Geometry: final body of the model. Coordinates: model frame, mm. A direction names the side the tool comes from. Round coordinates to 2 decimals unless told otherwise and drop trailing zeros. Write each loop counter-clockwise with the first axis right and the second up, starting at its lowest first coordinate (ties: lowest second). Pieces come first, ordered by that corner, then holes. Notation, with made-up numbers: M 75,37.5 L 128,37.5 A27 ccw 128,54.5 Z; hole C 47.25,42.25 d9. An arc over 180 degrees is marked long. Put each result on its own line as item: value. Start each with the question number.
```python
from build123d import *

# Parameters (mm, degrees)
SKETCH1_W            = 56
SKETCH1_H            = 199.6
EXTRUDE1_DEPTH       = 10
CHAMFER1_SIZE        = 1.5
HOLEWZD1_D           = 4
HOLEWZD1_DEPTH       = 5
HOLEWZD4_D           = 6.6
HOLEWZD4_DEPTH       = 10
HOLEWZD5_D           = 4
HOLEWZD5_DEPTH       = 10
HOLEWZD6_D           = 4
HOLEWZD6_DEPTH       = 5
HOLEWZD7_D           = 3.3
HOLEWZD9_D           = 4.5
HOLEWZD9_CBORE_D     = 8
HOLEWZD9_CBORE_DEPTH = 5


with BuildPart() as part:
    # Sketch1 → Extrude1 (new body)
    with BuildSketch(Plane.XY):
        with Locations((0, 78.3)):
            Rectangle(SKETCH1_W, SKETCH1_H)
    extrude(amount=EXTRUDE1_DEPTH)

    # Chamfer1
    chamfer1_edges = [part.edges().sort_by_distance(p)[0] for p in [
        (28, 78.3, 10),
        (0, 178.1, 10),
        (-28, 78.3, 10),
        (0, 178.1, 0),
        (28, 78.3, 0),
        (0, -21.5, 0),
        (-28, 78.3, 0),
        (0, -21.5, 10),
        (-28, 178.1, 5),
        (28, 178.1, 5),
        (28, -21.5, 5),
        (-28, -21.5, 5),
    ]]
    chamfer(chamfer1_edges, length=CHAMFER1_SIZE)

    # HoleWzd1
    with Locations(Plane(origin=(-28, 98.3, 0), x_dir=(-1, 0, 0), z_dir=(0, 0, -1))):
        with Locations((-40, -108.3), (-16, -108.3), (-40, 68.3), (-16, 68.3)):
            Hole(HOLEWZD1_D / 2, depth=HOLEWZD1_DEPTH)

    # HoleWzd4
    with Locations(Plane(origin=(0, 0, 0), x_dir=(-1, 0, 0), z_dir=(0, 0, -1))):
        with Locations((-12.5, 99.196924858), (12.5, 124.196924858), (-12.5, 124.196924858), (12.5, 99.196924858), (-12.5, 49.196924858), (12.5, 49.196924858), (12.5, 24.196924858), (-12.5, 24.196924858)):
            Hole(HOLEWZD4_D / 2, depth=HOLEWZD4_DEPTH)

    # HoleWzd5
    with Locations(Plane(origin=(0, 0, 0), x_dir=(-1, 0, 0), z_dir=(0, 0, -1))):
        with Locations((0, 111.696924858), (0, 36.696924858)):
            Hole(HOLEWZD5_D / 2, depth=HOLEWZD5_DEPTH)

    # HoleWzd6
    with Locations(Plane(origin=(0, 0, 0), x_dir=(-1, 0, 0), z_dir=(0, 0, -1))):
        with Locations((17.5, 88.301), (-17.5, 88.301)):
            Hole(HOLEWZD6_D / 2, depth=HOLEWZD6_DEPTH)

    # HoleWzd7 (through all)
    with Locations(Plane(origin=(0, 0, 0), x_dir=(-1, 0, 0), z_dir=(0, 0, -1))):
        with Locations((10, 88.301), (-10, 88.301)):
            Hole(HOLEWZD7_D / 2)

    # HoleWzd9 (through all)
    with Locations(Plane.XY.offset(10)):
        with Locations((20, -10), (-20, -10), (20, 166.6), (-20, 166.6)):
            CounterBoreHole(HOLEWZD9_D / 2, HOLEWZD9_CBORE_D / 2, HOLEWZD9_CBORE_DEPTH)


solid = part.part
```
1) Ray query, probe 1 along X at (y, z) = (124, 4.5); probe 2 along Y at (x, z) = (-20, 2.4); probe 3 along Y at (x, z) = (-15.5, 8.25). Return the intervals inside material, ascending.
2) Section A-A, the plane x = 0. Output: boundary loops of the cut face in (y, z), and give its area (3 significant figures).
3) First-contact query: pin 1 (2 mm diameter, centred on x = -12.5, y = -10, fed in from -Z); pin 2 (6.5 mm diameter, centred on x = 20, y = -10, fed in from +Z). Flat tips, straight axial feed; report the tip coordinate or a pass-through.
4) Access query for faces 1 (the face through (-10.4, 86.7, 5.1)), 2 (the face through (-23.2, -12.4, 7.5)), 3 (the face through (17, 88, 5)). Directions: +Z, -Z, +X, -X, +Y, -Y. A direction counts if a zero-diameter tool reaches every point of the face in a straight line with its end or side. Return the directions, or none.
5) Draft query along Y for faces 4 (the face through (10.07, 26.43, 5.07)), 5 (the face through (0, -21.5, 5)). Return one class per face: +Y half, -Y half, draft (parallel to the pull), parting line (faces both ways), or undercut.
Solved:
1. probe 1: x = -28 to -15.79, -9.21 to 9.21, 15.79 to 28
1. probe 2: y = -21.5 to -12.25, -7.75 to 164.35, 168.85 to 178.1
1. probe 3: y = -21.5 to 22.82, 25.57 to 47.82, 50.57 to 97.82, 100.57 to 122.82, 125.57 to 178.1
2. outline: M -21.5,1.5 L -20,0 L 34.7,0 L 34.7,10 L -20,10 L -21.5,8.5 Z; M 38.7,0 L 109.7,0 L 109.7,10 L 38.7,10 Z; M 113.7,0 L 176.6,0 L 178.1,1.5 L 178.1,8.5 L 176.6,10 L 113.7,10 Z
2. area: 1,910 mm2
3. pin 1: stops at z = 5
3. pin 2: stops at z = 5
4. face 1: +Z, -Z
4. face 2: +Z
4. face 3: -Z
5. face 4: undercut
5. face 5: -Y half
